Autodesk Fusion 360 part; units mm, degrees
sketch "草图1" plane through (0, 0, 0) normal (0, 0, 1) x (1, 0, 0)
  circle A0 centre (0, 0) radius 10
  circle A1 centre (0, 0) radius 3.275
  dimension "d1" = 20
  dimension "d2" = 6.55
extrude "拉伸1" add sketch "草图1" along normal blind 20
sketch "草图2" plane through (0, 0, 20) normal (0, 0, 1) x (-1, 0, 0)
  circle A0 centre (0, 0) radius 3.275
  circle A1 centre (0, 0) radius 10
  circle A2 centre (0, 0) radius 6
  dimension "d5" = 12
extrude "拉伸2" add sketch "草图2" along normal blind 50 contours A1
extrude "Extrude3" add 1 faces at (-5.0571, 0.4608, 20) along direction (0, 0, 1) blind 5
sketch "Sketch3" plane through (0, 0, 70) normal (0, 0, 1) x (-1, 0, 0)
  circle A0 centre (0, 0) radius 6
  circle A1 centre (0, 0) radius 10
  circle A2 centre (0, 0) radius 15
  dimension "d11" = 30
extrude "Extrude4" add sketch "Sketch3" against normal blind 70 contours A2
chamfer "Chamfer2" distance 5 angle 75 1 edges at (13.9849, -5.4242, 0) measured on face at (-11.0236, 0.9079, 0)
extrude "Extrude5" add 1 faces at (-11.9442, 0.7452, 70) along direction (0, 0, 1) blind 5
chamfer "Chamfer3" distance 0.5 angle 45 2 edges at (-3.0534, 1.1843, 25) (-3.0534, 1.1843, 0) 1 faces at (-11.9442, 0.7452, 75) measured on face at (-5.0571, 0.4608, 25) measured on face at (3.2709, -0.1632, 16.6667)
chamfer "Chamfer1" [suppressed]
Geometry: final body of the model. Coordinates: model frame, mm. A direction names the side the tool comes from. Round coordinates to 2 decimals unless told otherwise and drop trailing zeros. Order: outer loops, then holes, each group sorted by start corner. A loop starts at its lowest first (then second) coordinate and runs counter-clockwise, first axis right, second up. Notation, with made-up numbers: M -9.75,39.25 L 33.25,39.25 A12 cw 33.25,50.25 Z; hole C 66,-20.75 d9. An arc over 180 degrees is marked long. One line per item, written item: value.
(1) Pull-direction query (Y, two-part tool) for faces 3 (the cylindrical face through (6, 0, 49)), 4 (the cylindrical face through (14.985, -0.66, 46.971)), 5 (the flat face through (-4, 0, 0)); classes: pulls with the +Y half, pulls with the -Y half, needs draft (parallel to the pull), parting line crosses it, or undercut.
Result sheet:
face 3: undercut
face 4: parting line crosses it
face 5: needs draft
(2) Reachability of faces 1 (the flat face through (0, -4, 25)), 2 (the flat face through (-6, 3, 75)) from +Z, -Z, +X, -X, +Y, -Y: full face, straight path, thin tool, end or side. Return the list, or none.
Result sheet:
face 1: +Z
face 2: +Z, +X, -X, +Y, -Y
(3) Line query: probe 1 along Y at (x, z) = (0, 39); probe 2 along Y at (x, z) = (0, 18.75) (3 decimals). Output: solid intervals per line, ascending. Write a range as [from, to].
Result sheet:
probe 1: [-15, -6], [6, 15]
probe 2: [-15, -3.275], [3.275, 15]
(4) Pin query (flat end, axial travel): P1, Ø2, axis at x = -11.5, z = 33, coming from the +Y side; P2, Ø9.5, axis at x = 1.5, y = 2, coming from the +Z side; P3, Ø8, axis at x = 4.5, z = 16.5, coming from the +Y side; P4, Ø2, axis at y = -2, z = 20.5, coming from the +X side. Return the tip coordinate at first contact, or that it passes through.
Result sheet:
P1: y = 10.71
P2: z = 75
P3: y = 14.96
P4: x = 14.97
(5) Cut plane B-B (z = 53). Return the cut outline in (x, y), and give its area (3 significant figures).
Result sheet:
outline: C 0,0 d30; hole C 0,0 d12
area: 594 mm2
(6) Cut plane A-A (y = 0). Return the cut outline in (x, z) (3 decimals).
Result sheet:
outline: M -15,18.66 L -10,0 L -3.775,0 L -3.275,0.5 L -3.275,24.5 L -3.775,25 L -6,25 L -6,74.5 L -6.5,75 L -14.5,75 L -15,74.5 Z; M 3.275,0.5 L 3.775,0 L 10,0 L 15,18.66 L 15,74.5 L 14.5,75 L 6.5,75 L 6,74.5 L 6,25 L 3.775,25 L 3.275,24.5 Z
